Here's the drawing with two shaded views (mm, measured from the low corner). I have some questions. Round coordinates to 2 decimals unless told otherwise and drop trailing zeros. Order: outer loops, then holes, each group sorted by start corner. A loop starts at its lowest first (then second) coordinate and runs counter-clockwise, first axis right, second up.
Q1. Will these pins go through, and if not, where does the flat tip stop? P1, Ø1, axis at y = 20, z = 13, coming from the +X side; P2, Ø2, axis at x = 22.5, z = 7.5, coming from the +Y side; P3, Ø3.5, axis at x = 17.78, y = 2.54, coming from the +Z side; P4, Ø8, axis at x = 14.5, y = 24, coming from the -Z side.
Q2. If we section it at A-A (x = 17.78): Please give me the cut outline in (y, z).
Q3. We'd pull the mould along X, two halves only. Please class the marked faces 1, 2 and 3: pulls with the +X half, pulls with the -X half, needs draft (parallel to the pull), parting line crosses it, or undercut.
Q4. If we section it at C-C (x = 25.5): Please give me the cut outline in (y, z), plus the area to 3 significant figures.
Q5. If we section it at D-D (z = 15.25): Please give me the cut outline in (x, y) (1 decimal).
Q6. If we section it at B-B (y = 17.78): Please give me the cut outline in (x, z).
Q7. If I drill on line 1 (Y direction, x = 17.78, z = 0.3); line 2 (Y direction, x = 17.78, z = 16.25); line 3 (Z direction, x = 31.5, y = 21.5), over which ranges is the centre line in solid material (lowest first)?
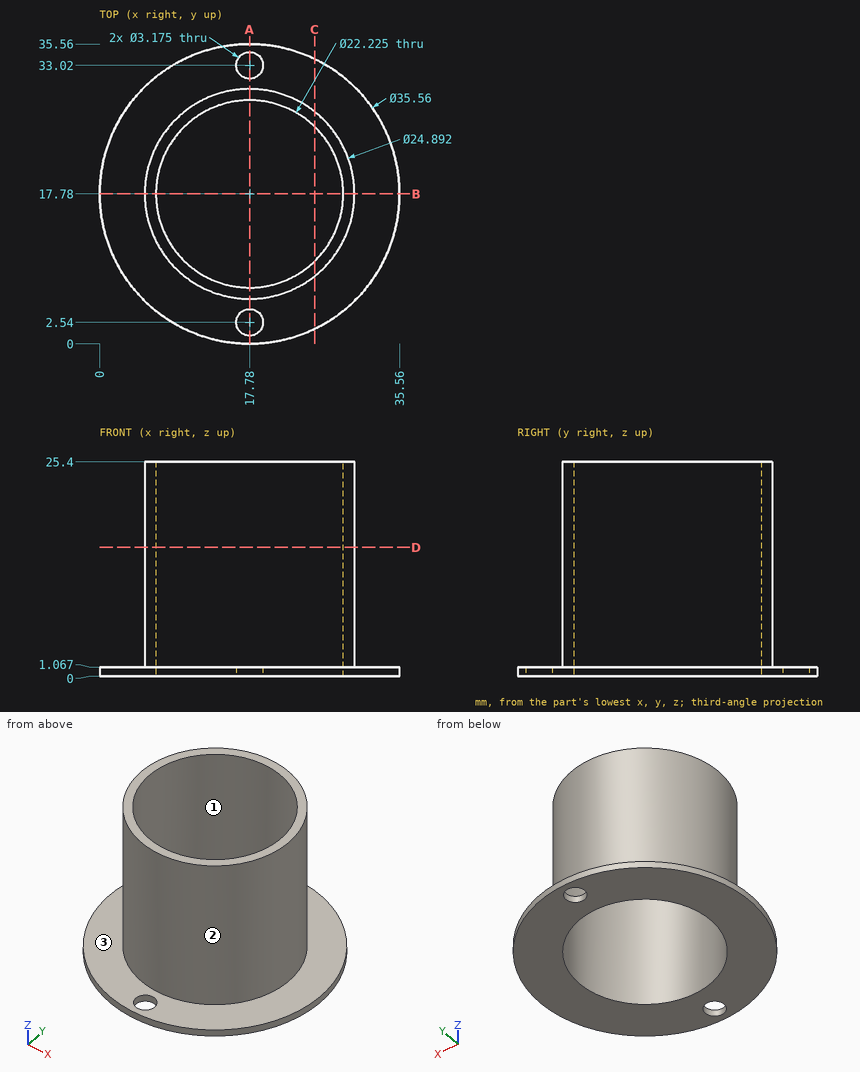
Solution:
1. P1: stops at x = 30.11
1. P2: stops at y = 29.66
1. P3: stops at z = 1.07
1. P4: passes through
2. outline: (0, 0) - (0.95, 0) - (0.95, 1.07) - (0, 1.07) - close; (4.13, 0) - (6.67, 0) - (6.67, 25.4) - (5.33, 25.4) - (5.33, 1.07) - (4.13, 1.07) - close; (28.89, 0) - (31.43, 0) - (31.43, 1.07) - (30.23, 1.07) - (30.23, 25.4) - (28.89, 25.4) - close; (34.61, 0) - (35.56, 0) - (35.56, 1.07) - (34.61, 1.07) - close
3. face 1: undercut
3. face 2: parting line crosses it
3. face 3: needs draft
4. outline: (1.76, 0) - (9.79, 0) - (9.79, 25.4) - (8.02, 25.4) - (8.02, 1.07) - (1.76, 1.07) - close; (25.77, 0) - (33.8, 0) - (33.8, 1.07) - (27.54, 1.07) - (27.54, 25.4) - (25.77, 25.4) - close
4. area: 103 mm2
5. outline: circle Ø24.9 at (17.8, 17.8); hole circle Ø22.2 at (17.8, 17.8)
6. outline: (0, 0) - (6.67, 0) - (6.67, 25.4) - (5.33, 25.4) - (5.33, 1.07) - (0, 1.07) - close; (28.89, 0) - (35.56, 0) - (35.56, 1.07) - (30.23, 1.07) - (30.23, 25.4) - (28.89, 25.4) - close
7. line 1: y = 0 to 0.95, 4.13 to 6.67, 28.89 to 31.43, 34.61 to 35.56
7. line 2: y = 5.33 to 6.67, 28.89 to 30.23
7. line 3: z = 0 to 1.07
